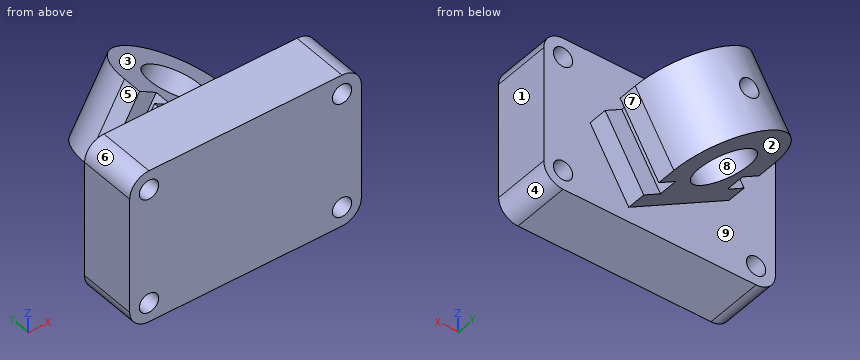
Autodesk Inventor part; units mm, degrees
sketch "Sketch1" plane through (0, 0, 0) normal (0, 1, 0) x (-1, 0, 0)
  line L0 (31.75, 25.4) -> (-31.75, 25.4)
  line L1 (-38.1, 19.05) -> (-38.1, -19.05)
  line L2 (-31.75, -25.4) -> (31.75, -25.4)
  line L3 (38.1, -19.05) -> (38.1, 19.05)
  arc A0 (31.75, -25.4) -> (38.1, -19.05) centre (31.75, -19.05) ccw
  arc A1 (38.1, 19.05) -> (31.75, 25.4) centre (31.75, 19.05) ccw
  arc A2 (-31.75, 25.4) -> (-38.1, 19.05) centre (-31.75, 19.05) ccw
  arc A3 (-38.1, -19.05) -> (-31.75, -25.4) centre (-31.75, -19.05) ccw
  circle A4 centre (31.75, -19.05) radius 3.175
  circle A5 centre (31.75, 19.05) radius 3.175
  circle A6 centre (-31.75, 19.05) radius 3.175
  circle A7 centre (-31.75, -19.05) radius 3.175
  point P0 (0, 0)
  dimension "d0" = 6.35
  dimension "d1" = 50.8
  dimension "d2" = 76.2
  dimension "d3" = 38.1
  dimension "d4" = 25.4
  dimension "d5" = 6.35
  dimension "d6" = 6.35
  dimension "d7" = 6.35
  dimension "d8" = 6.35
extrude "Extrusion1" add sketch "Sketch1" along normal blind 19.05
ref_plane "Work Plane1" through (0, 0, 0) normal (0.5, 0, 0.866) x (0, 1, 0)
sketch "Sketch2" plane through (0, 0, 0) normal (0.5, 0, 0.866) x (0, 1, 0)
  line L0 (19.05, -40.1963) -> (19.05, 14.7963)
  line L1 (0, 14.7963) -> (19.05, 14.7963)
  line L2 (25.3995, 19.0504) -> (25.3995, 12.7004)
  line L3 (25.3995, 12.7004) -> (31.7495, 12.7005)
  line L4 (31.7495, 12.7005) -> (31.7495, 19.0505)
  line L5 (31.7495, 19.0505) -> (38.0995, 19.0505)
  line L6 (38.1, -19.0495) -> (31.75, -19.0495)
  line L7 (31.75, -19.0495) -> (31.7499, -12.6995)
  line L8 (31.7499, -12.6995) -> (25.3999, -12.6996)
  line L9 (25.3999, -12.6996) -> (25.4, -19.0496)
  line L10 (19.05, -19.0497) -> (25.4, -19.0496)
  arc A0 (38.1, -19.0495) -> (38.0995, 19.0505) centre (38.1, 0.0005) ccw
  circle A1 centre (38.1, 0.0005) radius 9.525
  line L11 (25.3995, 19.0504) -> (19.05, 19.0504)
  line L12 (19.05, 19.0504) -> (19.05, -19.0497)
  point P0 (0, 0)
  dimension "d19" = 38.1
  dimension "d20" = 19.05
  dimension "d21" = 6.35
  dimension "d22" = 6.35
  dimension "d23" = 6.35
  dimension "d25" = 6.35
  dimension "d28" = 19.05
  dimension "d29" = 19.05
  dimension "d30" = 6.35
  dimension "d31" = 6.3495
  dimension "d32" = 38.1001
extrude "Extrusion2" add sketch "Sketch2" along normal mid plane 25.4
ref_plane "Work Plane2" through (0, 38.1, 0) normal (0, 1, 0) x (1, 0, 0)
sketch "Sketch3" plane through (0, 38.1, 0) normal (0, 1, 0) x (1, 0, 0)
  circle A0 centre (0, 0) radius 3.175
  dimension "d36" = 6.35
extrude "Extrusion3" cut sketch "Sketch3" along normal blind 25.4
equation "\"d6\" = d5"
equation "\"d7\" = d5"
equation "\"d8\" = d5"
properties part number "Chpt9_Tutorial"
The model under review builds one solid part; all positions refer to its coordinate system, in mm. Face numbers are marked on the shaded views. A direction names the side the tool comes from. Round coordinates to 2 decimals unless told otherwise and drop trailing zeros. Loops run counter-clockwise (first coordinate to the right, second up) from the corner with the lowest first, then second, coordinate; pieces in that order, holes last. Notation, with made-up numbers: (21.5, 34.5) - (53.5, 34.5) arc R6 cw to (53.5, 39.5) - close; hole circle Ø5 at (-23, 72). An arc over 180 degrees is marked (long way). Use CSV: the item, a comma, the result in double quotes.
(1) Take a section at A-A, the plane y = 13. Give the boundary of the cut face in (x, z) (3 decimals).
Working result:
outline,"(-38.1, -19.05) arc R6.35 ccw to (-31.75, -25.4) - (31.75, -25.4) arc R6.35 ccw to (38.1, -19.05) - (38.1, 19.05) arc R6.35 ccw to (31.75, 25.4) - (-31.75, 25.4) arc R6.35 ccw to (-38.1, 19.05) - close; hole circle Ø6.35 at (-31.75, -19.05); hole circle Ø6.35 at (-31.75, 19.05); hole circle Ø6.35 at (31.75, -19.05); hole circle Ø6.35 at (31.75, 19.05)"
(2) The part is to be moulded in two halves that separate along Z. For the marked faces 6, 7, 8 and 9, say which applies: pulls with the +Z half, pulls with the -Z half, needs draft (parallel to the pull), parting line crosses it, or undercut.
Working result:
face 6,"pulls with the +Z half"
face 7,"pulls with the -Z half"
face 8,"undercut"
face 9,"needs draft"
(3) Take a section at B-B, the plane y = 35.5. Give the boundary of the cut face in (x, z), plus the area to 3 significant figures.
Working result:
outline,"(-22.85, -1.47) - (-14.29, -6.42) - (-1.59, 15.58) - (-10.15, 20.52) - close; (1.59, -15.58) - (10.15, -20.52) - (22.85, 1.47) - (14.29, 6.42) - close"
area,"502 mm^2"
(4) Clearance check with flat-ended pins moving along their axes: P1, Ø20, axis at x = -11, z = 4.5, coming from the +Y side; P2, Ø5.5, axis at x = 31.75, z = -19.05, coming from the +Y side; P3, Ø1.5, axis at y = 39.5, z = 1, coming from the -X side; P4, Ø10, axis at x = 27.5, z = 8.5, coming from the +Y side. State where each tip first meets the part, or that it passes through.
Working result:
P1,"stops at y = 57.06"
P2,"passes through"
P3,"stops at x = -21.8"
P4,"stops at y = 19.05"
(5) Take a section at C-C, the plane y = 52. Give the boundary of the cut face in (x, z) (3 decimals).
Working result:
outline,"(-17.632, -4.485) - (4.931, -17.512) - (17.631, 4.485) - (-4.932, 17.512) - close; hole circle Ø6.35 at (0, 0)"
(6) Machinability: for the marked faces 1, 2, 3, 4 and 5, which of the approach directions +Z, -Z, +X, -X, +Y, -Y give a long, thin tool a straight path to every point of the face, cutting with its end or side? Answer none if there is none.
Working result:
face 1,"+Z, -Z, +X, +Y, -Y"
face 2,"-Z, -X, +Y"
face 3,"+Z, +X, +Y"
face 4,"-Z, +X, +Y, -Y"
face 5,"+Z, -X, +Y"
(7) For line 1 (X direction, y = 13, z = 19); line 2 (Z direction, x = 31, y = 4); line 3 (Y direction, x = -20, z = 17.5), list the stretches that pass through material, from the lowest coordinate up.
Working result:
line 1,"x = -38.1 to -34.92, -28.58 to 28.58, 34.92 to 38.1"
line 2,"z = -25.4 to -22.14, -15.96 to 15.96, 22.14 to 25.4"
line 3,"y = 0 to 19.05"
(8) Take a section at D-D, the plane x = 0. State how many separate pieces and enclosed holes the cut face has, plus the area to 3 significant figures.
Working result:
separate pieces,"3"
enclosed holes,"0"
area,"1,510 mm^2"
